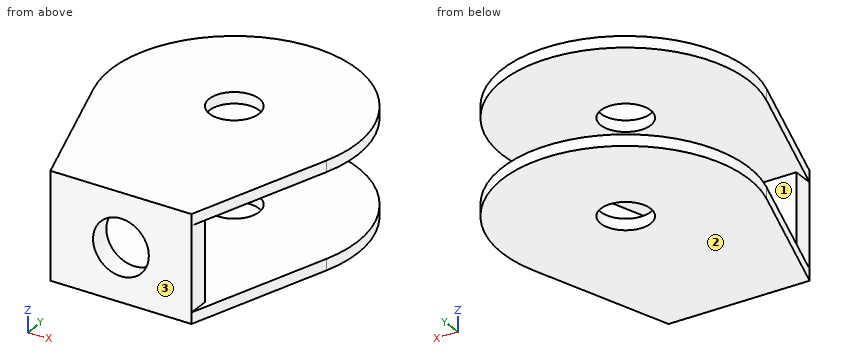
Autodesk Inventor part; units mm, degrees
ref_plane "YZ Plane" through (0, 0, 0) normal (1, 0, 0) x (0, 1, 0)
ref_plane "XZ Plane" through (0, 0, 0) normal (0, 1, 0) x (-1, 0, 0)
ref_plane "XY Plane" through (0, 0, 0) normal (0, 0, 1) x (1, 0, 0)
sketch "Sketch1" plane through (0, 0, 0) normal (0, 0, 1) x (1, 0, 0)
  line L0 (0, 0) -> (25.3, 0)
  line L1 (25.3, 0) -> (25.3, 16.2986) construction
  line L2 (25.3, 16.2986) -> (0, 16.2986) construction
  line L3 (0, 16.2986) -> (0, 0) construction
  circle A0 centre (12.65, 32) radius 4.45
  circle A1 centre (12.65, 32) radius 22
  line L4 (25.3, 0) -> (33.5525, 25.138)
  line L5 (0, 0) -> (-8.2525, 25.138)
  line L6 (12.65, 54) -> (12.65, 0)
  dimension "d0" = 25.3
  dimension "d1" = 8.9
  dimension "d2" = 32
  dimension "d3" = 44
  dimension "d16" = 12.65
extrude "Extrusion1" add sketch "Sketch1" along normal blind 2 contours L5 A1 L6 L0 | L6 A1 L4 L0 | A1 L6 A0 | L6 A0 A1
sketch "Sketch2" plane through (0, 0, 2) normal (0, 0, 1) x (1, 0, 0)
  line L0 (-8.2525, 25.138) -> (0, 0)
  line L1 (0, 0) -> (25.3, 0)
  line L2 (25.3, 0) -> (25.3, 3.75)
  line L3 (25.3, 3.75) -> (0, 3.75)
  line L4 (0, 3.75) -> (0, 0)
  dimension "d6" = 25.3
  dimension "d7" = 3.75
extrude "Extrusion2" add sketch "Sketch2" along normal blind 7.5
mirror "Mirror1" about plane through (12.65, 1.875, 9.5) normal (0, 0, 1) of "Extrusion1", "Extrusion2"
sketch "Sketch3" plane through (0, 0, 0) normal (0, -1, 0) x (1, 0, 0)
  line L0 (0, 0) -> (12.65, 0)
  line L1 (12.65, 0) -> (12.65, 9.5)
  line L2 (12.65, 9.5) -> (0, 9.5)
  line L3 (0, 9.5) -> (0, 0)
  circle A0 centre (12.65, 9.5) radius 5
  dimension "d10" = 9.5
  dimension "d11" = 12.65
  dimension "d12" = 10
extrude "Extrusion3" cut sketch "Sketch3" against normal blind 7.5 contours A0 L2 L1 | L1 L2 A0
properties part number "pulley"
Check sheet for the modelled part. Datum: model origin and axes. Units: mm. Face numbers are marked on the shaded views. Round coordinates to 2 decimals unless told otherwise and drop trailing zeros. Loops run counter-clockwise (first coordinate to the right, second up) from the corner with the lowest first, then second, coordinate; pieces in that order, holes last. Notation, with made-up numbers: M -32.5,-7 L 24.5,-7 A23 cw 24.5,18 Z; hole C 15.5,57.5 d9. An arc over 180 degrees is marked long. One line per item, written item: value.
(1) Release check for a two-part mould opening along Z. For the marked faces 1, 2 and 3 record: +Z half, -Z half, draft (parallel to the pull), parting line (faces both ways), or undercut.
Computed values:
face 1: undercut
face 2: -Z half
face 3: draft
(2) Depth check by flat-ended pin: pin 1 Ø1.1 at (y, z) = (3, 7) entering from -X; pin 2 Ø6 at (x, y) = (16, 30) entering from +Z; pin 3 Ø1.1 at (y, z) = (2.5, 10) entering from +X; pin 4 Ø4 at (y, z) = (12, 17) entering from -X. Enter the tip coordinate at first touch or a pass-through.
Computed values:
pin 1: stops at x = 0
pin 2: stops at z = 19
pin 3: stops at x = 25.3
pin 4: stops at x = -4.6
(3) Sectioned sample at B-B, the plane x = 12.65. Record the cut outline in (y, z), then the cut area to 3 significant figures.
Computed values:
outline: M 0,0 L 27.55,0 L 27.55,2 L 3.75,2 L 3.75,4.5 L 0,4.5 Z; M 0,14.5 L 3.75,14.5 L 3.75,17 L 27.55,17 L 27.55,19 L 0,19 Z; M 36.45,0 L 54,0 L 54,2 L 36.45,2 Z; M 36.45,17 L 54,17 L 54,19 L 36.45,19 Z
area: 199 mm^2
(4) Thickness scan on line 1 (Y direction, x = 12.65, z = 17.4); line 2 (Z direction, x = 6, y = 48); line 3 (X direction, y = 2.95, z = 9.5). Record the ranges inside material, lowest first.
Computed values:
line 1: y = 0 to 27.55, 36.45 to 54
line 2: z = 0 to 2, 17 to 19
line 3: x = 0 to 7.65, 17.65 to 25.3
(5) Sectioned sample at C-C, the plane y = 32. Record the cut outline in (x, z).
Computed values:
outline: M -9.35,0 L 8.2,0 L 8.2,2 L -9.35,2 Z; M -9.35,17 L 8.2,17 L 8.2,19 L -9.35,19 Z; M 17.1,0 L 34.65,0 L 34.65,2 L 17.1,2 Z; M 17.1,17 L 34.65,17 L 34.65,19 L 17.1,19 Z
(6) Sectioned sample at D-D, the plane y = 46. Record the cut outline in (x, z).
Computed values:
outline: M -4.32,0 L 29.62,0 L 29.62,2 L -4.32,2 Z; M -4.32,17 L 29.62,17 L 29.62,19 L -4.32,19 Z
(7) Sectioned sample at A-A, the plane z = 9.5. Record the cut outline in (x, y), then the cut area to 3 significant figures.
Computed values:
outline: M 0,0 L 7.65,0 L 7.65,3.75 L 0,3.75 Z; M 17.65,0 L 25.3,0 L 25.3,3.75 L 17.65,3.75 Z
area: 57.4 mm^2
